```python
from build123d import *

# Parameters (mm, degrees)
SKETCH1_W           = 56
SKETCH1_H           = 19.7
BOSS_EXTRUDE2_DEPTH = 11
SKETCH3_W           = 60
SKETCH3_H           = 23.7
BOSS_EXTRUDE3_DEPTH = 1
SKETCH4_R           = 8.25
CUT_EXTRUDE1_DEPTH  = 35.415439849
CUT_EXTRUDE2_DEPTH  = 5
FILLET1_R           = 2
CUT_EXTRUDE3_DEPTH  = 5
FILLET2_R           = 2


with BuildPart() as part:
    # Sketch1 → Boss-Extrude2 (new body)
    with BuildSketch(Plane.XY):
        Rectangle(SKETCH1_W, SKETCH1_H)
    extrude(amount=BOSS_EXTRUDE2_DEPTH)

    # Sketch3 → Boss-Extrude3 (add)
    with BuildSketch(Plane.XY.offset(11)):
        Rectangle(SKETCH3_W, SKETCH3_H)
    extrude(amount=BOSS_EXTRUDE3_DEPTH)

    # Sketch4 → Cut-Extrude1 (cut, through all)
    with BuildSketch(Plane.XY.offset(12)):
        with Locations((-12.75, 0)):
            Circle(SKETCH4_R)
        with Locations((12.75, 0)):
            Circle(SKETCH4_R)
    extrude(amount=-CUT_EXTRUDE1_DEPTH, mode=Mode.SUBTRACT)

    # Sketch5 → Cut-Extrude2 (cut)
    with BuildSketch(Plane(origin=(0, 0, 0), x_dir=(-1, 0, 0), z_dir=(0, 0, -1))):
        with BuildLine():
            Line((-5.75, 9.85), (5.75, 9.85))
            Line((5.75, 9.85), (5.75, 6.85))
            ThreePointArc((5.75, 6.85), (5.164213562, 5.435786438), (3.75, 4.85))
            Line((3.75, 4.85), (-3.75, 4.85))
            ThreePointArc((-3.75, 4.85), (-5.164213562, 5.435786438), (-5.75, 6.85))
            Line((-5.75, 6.85), (-5.75, 9.85))
        make_face()
    extrude(amount=-CUT_EXTRUDE2_DEPTH, mode=Mode.SUBTRACT)

    # Fillet1
    fillet1_edges = [part.edges().sort_by_distance(p)[0] for p in [
        (5.75, 9.85, 2.5),
        (-5.75, 9.85, 2.5),
    ]]
    fillet(fillet1_edges, radius=FILLET1_R)

    # Sketch6 → Cut-Extrude3 (cut)
    with BuildSketch(Plane(origin=(0, 0, 0), x_dir=(-1, 0, 0), z_dir=(0, 0, -1))):
        with BuildLine():
            Line((-3.75, -4.85), (3.75, -4.85))
            ThreePointArc((3.75, -4.85), (5.164213562, -5.435786438), (5.75, -6.85))
            Line((5.75, -6.85), (5.75, -9.85))
            Line((5.75, -9.85), (-5.75, -9.85))
            Line((-5.75, -9.85), (-5.75, -6.85))
            ThreePointArc((-5.75, -6.85), (-5.164213562, -5.435786438), (-3.75, -4.85))
        make_face()
    extrude(amount=-CUT_EXTRUDE3_DEPTH, mode=Mode.SUBTRACT)

    # Fillet2
    fillet2_edges = [part.edges().sort_by_distance(p)[0] for p in [
        (-5.75, -9.85, 2.5),
        (5.75, -9.85, 2.5),
    ]]
    fillet(fillet2_edges, radius=FILLET2_R)


solid = part.part
```
Part model, mm, in its own coordinate system. A direction names the side the tool comes from. Give positions to 0.01 mm unless a question says otherwise; leave off trailing zeros. Write each loop counter-clockwise with the first axis right and the second up, starting at its lowest first coordinate (ties: lowest second). Pieces come first, ordered by that corner, then holes. Notation, with made-up numbers: M 59.25,22 L 93.25,22 A30 cw 93.25,53 Z; hole C 53,15 d2. An arc over 180 degrees is marked long. Use CSV: the item, a comma, the result in double quotes.
Item 1: Pull direction X, two halves, no side cores. Call faces 4 (the face through (5.18, -5.45, 2.46)), 5 (the face through (-4.88, 2.48, 6.08)), 6 (the face through (0, 0, 12)), 7 (the face through (28, 0, 5)): +X half, -X half, draft (parallel to the pull), parting line (faces both ways), or undercut.
Taken from the geometry:
face 4,"undercut"
face 5,"undercut"
face 6,"draft"
face 7,"+X half"
Item 2: Which spindle directions (+Z, -Z, +X, -X, +Y, -Y) get a long thin tool onto all of the face, cutting with end or side? Do faces 1 (the face through (-0.4, -9.85, 5.4)), 2 (the face through (0, 4.85, 2)), 3 (the face through (-6.35, -9.28, 2.54)). Say none if no direction does.
Taken from the geometry:
face 1,"-Z, +X, -X, -Y"
face 2,"-Z, +Y"
face 3,"-Z, -Y"
Item 3: Drill centre lines: probe 1 along Y at (x, z) = (12.75, 9); probe 2 along X at (y, z) = (-5.75, 9.25); probe 3 along X at (y, z) = (2.75, 5.5). Where is each one in solid material? Low to high.
Taken from the geometry:
probe 1,"y = -9.85 to -8.25, 8.25 to 9.85"
probe 2,"x = -28 to -18.67, -6.83 to 6.83, 18.67 to 28"
probe 3,"x = -28 to -20.53, -4.97 to 4.97, 20.53 to 28"
Item 4: Slice it at C-C on y = 3.75. Write the cut outline in (x, z).
Taken from the geometry:
outline,"M -30,11 L -28,11 L -28,0 L -20.1,0 L -20.1,12 L -30,12 Z; M -5.4,0 L 5.4,0 L 5.4,12 L -5.4,12 Z; M 20.1,0 L 28,0 L 28,11 L 30,11 L 30,12 L 20.1,12 Z"
Item 5: Slice it at D-D on x = 0. Write the cut outline in (y, z).
Taken from the geometry:
outline,"M -11.85,11 L -9.85,11 L -9.85,5 L -4.85,5 L -4.85,0 L 4.85,0 L 4.85,5 L 9.85,5 L 9.85,11 L 11.85,11 L 11.85,12 L -11.85,12 Z"
Item 6: Slice it at B-B on z = 9.5. Write the cut outline in (x, y).
Taken from the geometry:
outline,"M -28,-9.85 L 28,-9.85 L 28,9.85 L -28,9.85 Z; hole C -12.75,0 d16.5; hole C 12.75,0 d16.5"
Item 7: Slice it at A-A on x = -12.75. Write the cut outline in (y, z).
Taken from the geometry:
outline,"M -11.85,11 L -9.85,11 L -9.85,0 L -8.25,0 L -8.25,12 L -11.85,12 Z; M 8.25,0 L 9.85,0 L 9.85,11 L 11.85,11 L 11.85,12 L 8.25,12 Z"
Item 8: Pin check, flat tips, straight feed: P1, Ø4, axis at x = -1.5, y = 8.5, coming from the -Z side; P2, Ø5.5, axis at x = -1, z = 3, coming from the +Y side; P3, Ø5, axis at y = 7.5, z = 2, coming from the +X side. Stop position of each tip, or through.
Taken from the geometry:
P1,"stops at z = 5"
P2,"stops at y = 9.85"
P3,"stops at x = 28"
